Source: CAD feature listing. Evaluate the final solid. Frame: model axes, mm. A direction names the side the tool comes from. Round coordinates to 2 decimals unless told otherwise and drop trailing zeros. Loops run counter-clockwise (first coordinate to the right, second up) from the corner with the lowest first, then second, coordinate; pieces in that order, holes last.
(1) Mould query, pull axis Z, two halves, no side actions, for faces 1 (the cylindrical face through (45.432, 18.044, 21.854)), 2 (the flat face through (-20, 22.1, -8)), 3 (the flat face through (-3.5, 21, -8)). Classes: pulls with the +Z half, pulls with the -Z half, needs draft (parallel to the pull), parting line crosses it, or undercut.
(2) Set-up query: faces 4 (the flat face through (6.5, 21, -8)), 5 (the cylindrical face through (44.93, 17.14, -36.63)), 6 (the cylindrical face through (-44.038, 18.044, 21.799)), 7 (the cylindrical face through (-44.543, 18.649, 5.052)). Return all of +Z, -Z, +X, -X, +Y, -Y with unobstructed straight access to the full face (end or side cutting, diameter ignored); none if empty.
(3) Section C-C, the plane z = -22.5. Count the separate pieces of the cut face and the enclosed holes in it, plus the area to 3 significant figures.
(4) Section A-A, the plane x = 10.5. Return the cut outline in (y, z), plus the area to 3 significant figures.
(5) Material intervals for probe 1 along X at (y, z) = (18, -34); probe 2 along Z at (x, y) = (-31, 17.25); probe 3 along X at (y, z) = (18.75, 10), sorted ascending.
(6) Section B-B, the plane x = -7. Return the cut outline in (y, z).
(7) First-contact query: pin 1 Ø2 at (x, z) = (-5.5, -7) entering from -Y; pin 2 Ø1.1 at (x, y) = (-44.5, 16) entering from -Z; pin 3 Ø1.1 at (x, y) = (-44.5, 15.5) entering from +Z. Flat tips, straight axial feed; report the tip coordinate or a pass-through.
```python
from build123d import *

# Parameters (mm, degrees)
SKETCH1_W           = 91.55
SKETCH1_H           = 61.1
BOSS_EXTRUDE1_DEPTH = 8
SKETCH2_W           = 89.55
SKETCH2_H           = 59.1
CUT_EXTRUDE1_DEPTH  = 6
CUT_EXTRUDE2_REACH  = 189.594
SKETCH3_W           = 13.7
SKETCH3_H           = 5.15
CUT_EXTRUDE3_REACH  = 189.594
SKETCH4_W           = 13.7
SKETCH4_H           = 5.15
CUT_EXTRUDE4_REACH  = 189.594
FILLET1_R           = 2
FILLET2_R           = 3.55
CUT_EXTRUDE5_DEPTH  = 2
LPATTERN1_COUNT     = 10
LPATTERN1_PITCH     = 5


with BuildPart() as part:
    # Sketch1 → Boss-Extrude1 (new body)
    with BuildSketch(Plane(origin=(0, 22.1, -139.373711609), x_dir=(1, 0, 0), z_dir=(0, 1, 0))):
        with Locations((0.725, -131.69)):
            Rectangle(SKETCH1_W, SKETCH1_H)
    extrude(amount=-BOSS_EXTRUDE1_DEPTH)

    # Sketch2 → Cut-Extrude1 (cut)
    with BuildSketch(Plane(origin=(0, 14.1, -139.373711609), x_dir=(1, 0, 0), z_dir=(0, -1, 0))):
        with Locations((0.725, 131.69)):
            Rectangle(SKETCH2_W, SKETCH2_H)
    extrude(amount=-CUT_EXTRUDE1_DEPTH, mode=Mode.SUBTRACT)

    # Sketch3 → Cut-Extrude2 (cut, up to next)
    with BuildSketch(Plane(origin=(-45.05, 0, -139.373711609), x_dir=(0, 0, 1), z_dir=(-1, 0, 0)), mode=Mode.PRIVATE) as cut_extrude2_sk1:
        with Locations((150.705690784, 16.675)):
            Rectangle(SKETCH3_W, SKETCH3_H)
    cut_extrude2_tool1 = extrude(cut_extrude2_sk1.sketch, amount=-CUT_EXTRUDE2_REACH, mode=Mode.PRIVATE) & part.part
    add(cut_extrude2_tool1.solids().sort_by_distance((-45.05, 16.675, 11.331979))[0], mode=Mode.SUBTRACT)

    # Sketch4 → Cut-Extrude3 (cut, up to next)
    with BuildSketch(Plane(origin=(-45.05, 0, -139.373711609), x_dir=(0, 0, 1), z_dir=(-1, 0, 0)), mode=Mode.PRIVATE) as cut_extrude3_sk1:
        with Locations((132.305690784, 16.675)):
            Rectangle(SKETCH4_W, SKETCH4_H)
    cut_extrude3_tool1 = extrude(cut_extrude3_sk1.sketch, amount=-CUT_EXTRUDE3_REACH, mode=Mode.PRIVATE) & part.part
    add(cut_extrude3_tool1.solids().sort_by_distance((-45.05, 16.675, -7.068021))[0], mode=Mode.SUBTRACT)

    # Sketch5 → Cut-Extrude4 (cut, up to next)
    with BuildSketch(Plane(origin=(-45.05, 0, -139.373711609), x_dir=(0, 0, 1), z_dir=(-1, 0, 0)), mode=Mode.PRIVATE) as cut_extrude4_sk1:
        with BuildLine():
            Line((106.718199777, 14.1), (120.891183123, 14.1))
            ThreePointArc((120.891183123, 14.1), (120.179436321, 15.18113883), (118.95469145, 15.6))
            Line((118.95469145, 15.6), (108.65469145, 15.6))
            ThreePointArc((108.65469145, 15.6), (107.429946578, 15.18113883), (106.718199777, 14.1))
        make_face()
    cut_extrude4_tool1 = extrude(cut_extrude4_sk1.sketch, amount=-CUT_EXTRUDE4_REACH, mode=Mode.PRIVATE) & part.part
    add(cut_extrude4_tool1.solids().sort_by_distance((-45.05, 14.822712, -25.56902))[0], mode=Mode.SUBTRACT)

    # Fillet1
    fillet1_edges = [part.edges().sort_by_distance(p)[0] for p in [
        (-44.05, 17.1, 21.866288391),
        (45.5, 17.1, 21.866288391),
        (45.5, 17.1, -37.233711609),
        (-44.05, 17.1, -37.233711609),
        (-44.55, 19.25, 18.181979175),
        (-44.55, 19.25, 4.481979175),
        (-44.55, 19.25, -0.218020825),
        (-44.55, 19.25, -13.918020825),
    ]]
    fillet(fillet1_edges, radius=FILLET1_R)

    # Fillet2
    fillet2_edges = [part.edges().sort_by_distance(p)[0] for p in [
        (-45.05, 18.1, 22.866288391),
        (-45.05, 18.1, -38.233711609),
        (46.5, 18.1, -38.233711609),
        (46.5, 18.1, 22.866288391),
    ]]
    fillet(fillet2_edges, radius=FILLET2_R)

    # Sketch6 → Cut-Extrude5 (cut)
    with BuildSketch(Plane(origin=(0, 22.1, 0), x_dir=(1, 0, 0), z_dir=(0, 1, 0))):
        with BuildLine():
            Line((36.5, 31.233711609), (36.5, -15.866288391))
            ThreePointArc((36.5, -15.866288391), (35.5, -16.866288391), (34.5, -15.866288391))
            Line((34.5, -15.866288391), (34.5, 31.233711609))
            ThreePointArc((34.5, 31.233711609), (35.5, 32.233711609), (36.5, 31.233711609))
        make_face()
    cut_extrude5 = extrude(amount=-CUT_EXTRUDE5_DEPTH, mode=Mode.SUBTRACT)

    # LPattern1: Cut-Extrude5 ×10
    with Locations(*[(-i * LPATTERN1_PITCH, 0, 0) for i in range(1, LPATTERN1_COUNT)]):
        add(cut_extrude5, mode=Mode.SUBTRACT)


solid = part.part
```
Output values:
1. face 1: pulls with the +Z half
1. face 2: needs draft
1. face 3: undercut
2. face 4: +Y, -Y
2. face 5: -Y
2. face 6: +Z, -X, +Y, -Y
2. face 7: -X, -Y
3. separate pieces: 11
3. enclosed holes: 0
3. area: 154 mm2
4. outline: (14.1, -38.23) - (22.1, -38.23) - (22.1, -32.23) - (20.1, -32.23) - (20.1, -37.23) - (14.1, -37.23) - close; (14.1, 21.87) - (20.1, 21.87) - (20.1, 16.87) - (22.1, 16.87) - (22.1, 22.87) - (14.1, 22.87) - close
4. area: 36.0 mm2
5. probe 1: x = -45.05 to -44.05, 45.5 to 46.5
5. probe 2: z = -38.23 to -37.23, 21.87 to 22.87
5. probe 3: x = 45.5 to 46.5
6. outline: (14.1, -38.23) - (22.1, -38.23) - (22.1, 22.87) - (14.1, 22.87) - (14.1, 21.87) - (20.1, 21.87) - (20.1, -37.23) - (14.1, -37.23) - close
7. pin 1: stops at y = 20.1
7. pin 2: stops at z = -37.25
7. pin 3: stops at z = 21.89
